from build123d import *

# Parameters (mm, degrees)
F0_R     = 114.3
F1_DEPTH = 9.525
F2_R     = 2.15265
F3_DEPTH = 3.175
F4_R     = 2.15265
F5_DEPTH = 3.175


with BuildPart() as f1:
    # F0 (on Top) → F1 (new body)
    with BuildSketch(Plane.XY):
        Circle(F0_R)
    extrude(amount=F1_DEPTH)

    # F2 (on face) → F3 (cut)
    with BuildSketch(Plane.XY.offset(9.525)):
        with Locations((-76.332177, 76.332177)):
            Circle(F2_R)
        with Locations((76.332177, 76.332177)):
            Circle(F2_R)
        with Locations((76.332177, -76.332177)):
            Circle(F2_R)
        with Locations((-76.332177, -76.332177)):
            Circle(F2_R)
    extrude(amount=-F3_DEPTH, mode=Mode.SUBTRACT)

    # F4 (on face) → F5 (cut)
    with BuildSketch(Plane(origin=(0, 0, 0), x_dir=(1, 0, 0), z_dir=(0, 0, -1))):
        with Locations((-76.332177, 76.332177)):
            Circle(F4_R)
        with Locations((76.332177, 76.332177)):
            Circle(F4_R)
        with Locations((76.332177, -76.332177)):
            Circle(F4_R)
        with Locations((-76.332177, -76.332177)):
            Circle(F4_R)
    extrude(amount=-F5_DEPTH, mode=Mode.SUBTRACT)


solid = f1.part
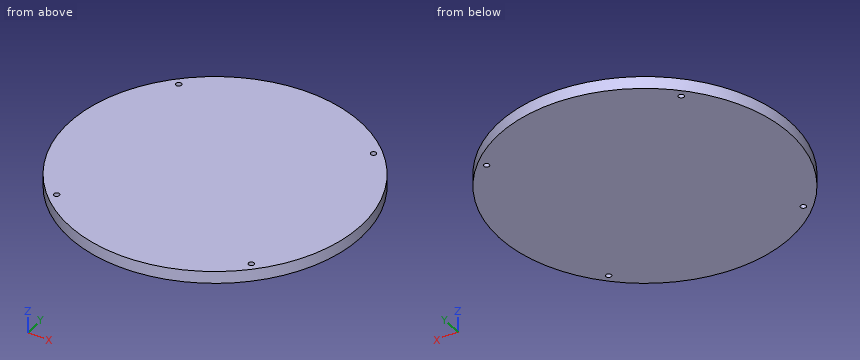
The listing builds one solid part. Answer for the finished solid, in the listing's coordinates (mm). Round coordinates to 2 decimals unless told otherwise and drop trailing zeros. Order: outer loops, then holes, each group sorted by start corner. A loop starts at its lowest first (then second) coordinate and runs counter-clockwise, first axis right, second up. Notation, with made-up numbers: (12.25, 19) -> (57.25, 19) arc R14 cw to (57.25, 41) -> close; hole circle Ø11 at (35.5, 54.5). An arc over 180 degrees is marked (long way). Write each question's results on one line, items separated by ' | '. Start each with the question number.
Q1. Straight lines are drawn through the part: probe 1 along Z at (x, y) = (-75.5, 76) (3 decimals); probe 2 along X at (y, z) = (-75, 4.5); probe 3 along Y at (x, z) = (34, 3.5). For each, find the intervals that lie inside material, in ascending order. Write a range as from..to.
Q2. Each of these flat-tipped pins is pushed along its axis until it touches: pin 1 (1.5 mm diameter, centred on x = -25.5, z = 4.5, fed in from +Y); pin 2 (4.5 mm diameter, centred on x = 75.5, y = -77.5, fed in from +Z) (3 decimals); pin 3 (1.3 mm diameter, centred on x = -76, y = -75.5, fed in from -Z) (3 decimals); pin 4 (2 mm diameter, centred on x = 76, y = 77, fed in from +Z). Where does it stop, or does it pass through?
Q3. Find section A-A (z = 8). Determine the outline of the cut face in (x, y), then the cut area to 3 significant figures.
Q4. Find section B-B (x = -36.5). Determine the outline of the cut face in (y, z) (3 decimals), then the cut area to 3 significant figures.
Q5. Find section C-C (y = -41.5). Determine the outline of the cut face in (x, z) (3 decimals), then the cut area to 3 significant figures.
Worked answers:
1) probe 1: z = 3.175..6.35 | probe 2: x = -86.25..86.25 | probe 3: y = -109.13..109.13
2) pin 1: stops at y = 111.59 | pin 2: stops at z = 9.525 | pin 3: stops at z = 3.175 | pin 4: stops at z = 6.35
3) outline: circle Ø228.6 at (0, 0); hole circle Ø4.31 at (-76.33, -76.33); hole circle Ø4.31 at (-76.33, 76.33); hole circle Ø4.31 at (76.33, -76.33); hole circle Ø4.31 at (76.33, 76.33) | area: 41,000 mm2
4) outline: (-108.315, 0) -> (108.315, 0) -> (108.315, 9.525) -> (-108.315, 9.525) -> close | area: 2,060 mm2
5) outline: (-106.5, 0) -> (106.5, 0) -> (106.5, 9.525) -> (-106.5, 9.525) -> close | area: 2,030 mm2
